The listing builds one solid part. Answer for the finished solid, in the listing's coordinates (mm). Round coordinates to 2 decimals unless told otherwise and drop trailing zeros. Write each loop counter-clockwise with the first axis right and the second up, starting at its lowest first coordinate (ties: lowest second). Pieces come first, ordered by that corner, then holes.
(1) Find the intervals of material crossed by probe 1 along X at (y, z) = (-106.5, 0.3); probe 2 along Y at (x, z) = (120, 1.25); probe 3 along X at (y, z) = (3.5, 0.4), in increasing order.
(2) A cutting plane is placed at A-A, the plane x = -2. Give the vertices of the cut face in (y, z).
(3) A cutting plane is placed at B-B, the plane z = 0.6. Give the number of separate pieces and of enclosed holes in the cut face, and give its area (3 significant figures).
Autodesk Inventor part; units mm, degrees
ref_plane "YZ Plane" through (0, 0, 0) normal (1, 0, 0) x (0, 1, 0)
ref_plane "XZ Plane" through (0, 0, 0) normal (0, 1, 0) x (-1, 0, 0)
ref_plane "XY Plane" through (0, 0, 0) normal (0, 0, 1) x (1, 0, 0)
sketch "Эскиз1" plane through (0, 0, 0) normal (0, 0, 1) x (1, 0, 0)
  line L0 (-145, 120) -> (145, 120)
  line L1 (145, 120) -> (145, -120)
  line L2 (145, -120) -> (-145, -120)
  line L3 (-145, -120) -> (-145, 120)
  line L4 (-145, 120) -> (145, -120) construction
  line L5 (145, 120) -> (-145, -120) construction
  point P0 (0, 0)
  dimension "d0" = 290
  dimension "d1" = 240
extrude "Выдавливание1" add sketch "Эскиз1" along normal blind 3
sketch "Эскиз2" plane through (0, 0, 3) normal (0, 0, 1) x (1, 0, 0)
  line L0 (-5, 95) -> (5, 95)
  line L1 (145, 120) -> (-145, 120)
  line L2 (0, 168) -> (0, -168)
  line L3 (-101.423, -89.3301) -> (-106.423, -80.6699)
  line L4 (106.423, -80.6699) -> (101.423, -89.3301)
  point P0 (0, 0)
  point P1 (0, 95)
  point P2 (0, -25)
  point P3 (-103.923, -85)
  point P4 (103.923, -85)
  dimension "d4" = 25
  dimension "d5" = 10
  dimension "d8" = 360
  dimension "d10" = 120
sketch "Эскиз4" plane through (0, 0, 0) normal (0, 0, -1) x (-1, 0, 0)
  line L0 (130, -15.5) -> (130, 9.5)
  line L1 (130, 9.5) -> (140, 9.5)
  line L2 (140, 9.5) -> (140, -15.5)
  line L3 (140, -15.5) -> (130, -15.5)
  line L4 (-15, -100) -> (15, -100)
  line L5 (15, -100) -> (15, -110)
  line L6 (15, -110) -> (-15, -110)
  line L7 (-15, -110) -> (-15, -100)
  line L8 (115, -100) -> (115, -110)
  line L9 (115, -110) -> (85, -110)
  line L10 (85, -110) -> (85, -100)
  line L11 (85, -100) -> (115, -100)
  line L12 (-130, -15.5) -> (-140, -15.5)
  line L13 (-140, -15.5) -> (-140, 9.5)
  line L14 (-140, 9.5) -> (-130, 9.5)
  line L15 (-130, 9.5) -> (-130, -15.5)
  circle A0 centre (120, 79) radius 1.5
  circle A1 centre (-120, -85) radius 1.5
  circle A2 centre (120, -85) radius 1.5
  line L16 (-85, -100) -> (-85, -110)
  line L17 (-85, -110) -> (-115, -110)
  line L18 (-115, -110) -> (-115, -100)
  line L19 (-115, -100) -> (-85, -100)
  circle A3 centre (-120, 79) radius 1.5
  line L20 (150, 119) -> (-150, 119)
  line L21 (-150, 119) -> (-150, -125)
  line L22 (-150, -125) -> (150, -125)
  line L23 (150, -125) -> (150, 119)
  point P0 (0, 0)
extrude "Выдавливание3" cut sketch "Эскиз4" against normal blind 10 contours L0 L1 L2 L3 | L4 L5 L6 L7 | L8 L9 L10 L11 | L12 L13 L14 L15 | A0 | A1 | A2 | L16 L17 L18 L19 | A3
sketch "Эскиз6" plane through (0, 0, 0) normal (0, 0, -1) x (-1, 0, 0)
  circle A0 centre (-115.363, -29) radius 2.5
  circle A1 centre (-115.363, 29) radius 2.5
  circle A2 centre (-74.363, 29) radius 2.5
  circle A3 centre (-74.363, -29) radius 2.5
  circle A4 centre (-25.5005, 12.1735) radius 1.0922
  circle A5 centre (-33.1205, 7.0935) radius 1.0922
  circle A6 centre (-25.5005, 12.1735) radius 1.0922
  circle A7 centre (16.1281, -25.2259) radius 1.5
  circle A8 centre (16.1281, -52.2259) radius 1.5
  circle A9 centre (-13.4032, -52.2259) radius 1.5
  circle A10 centre (-13.4032, -25.2259) radius 1.5
  circle A11 centre (66.1296, 35.3961) radius 1.5875
  circle A12 centre (66.1296, -47.1539) radius 1.5875
  circle A13 centre (114.3896, -40.8039) radius 1.5875
  circle A14 centre (99.1496, -16.6739) radius 1.5875
  circle A15 centre (71.2096, -16.6739) radius 1.5875
  circle A16 centre (114.3896, 34.1261) radius 1.5875
  line L0 (30, 37.5) -> (33, 37.5)
  line L1 (30, 34.5) -> (33, 34.5)
  line L2 (-33, 37.5) -> (-30, 37.5)
  line L3 (-33, 34.5) -> (-30, 34.5)
  line L4 (-33, 78.5) -> (-30, 78.5)
  line L5 (-33, 81.5) -> (-30, 81.5)
  line L6 (30, 78.5) -> (33, 78.5)
  line L7 (30, 81.5) -> (33, 81.5)
  circle A17 centre (31.5, 36) radius 1.5
  line L8 (33, 34.5) -> (33, 37.5) construction
  line L9 (-30, 34.5) -> (-30, 37.5) construction
  circle A18 centre (-31.5, 36) radius 1.5
  line L10 (33, 78.5) -> (33, 81.5) construction
  circle A19 centre (31.5, 80) radius 1.5
  circle A20 centre (-31.5, 80) radius 1.5
  line L11 (-33, 78.5) -> (-33, 81.5) construction
  point P0 (0, 0)
  dimension "d18" = 3
extrude "Выдавливание4" cut sketch "Эскиз6" against normal blind 10
sketch "Эскиз7" plane through (0, 0, 0) normal (0, 0, -1) x (-1, 0, 0)
  circle A0 centre (-95, 80) radius 1.5
  circle A1 centre (95, 80) radius 1.5
  circle A2 centre (95, -80) radius 1.5
  circle A3 centre (-95, -80) radius 1.5
  line L0 (-95, 80) -> (95, 80) construction
  line L1 (95, -80) -> (95, 80) construction
  circle A4 centre (-120, -85) radius 1.5 construction
  line L2 (-95, -80) -> (95, -80) construction
  line L3 (145, -120) -> (-145, -120) construction
  line L4 (-145, 120) -> (145, 120) construction
  line L5 (145, 120) -> (145, -120) construction
  line L6 (-95, 80) -> (-95, -80) construction
  line L7 (-145, -120) -> (-145, 120) construction
  point P0 (0, 0)
  dimension "d19" = 40
  dimension "d20" = 40
  dimension "d21" = 50
  dimension "d22" = 50
  dimension "d23" = 3
extrude "Выдавливание5" cut sketch "Эскиз7" against normal blind 10
properties part number "electronic_plate_long_side"
Solutions:
1. probe 1: x = -145 to -115, -85 to -15, 15 to 85, 115 to 145
1. probe 2: y = -120 to -86.5, -83.5 to 77.5, 80.5 to 120
1. probe 3: x = -145 to -140, -130 to 130, 140 to 145
2. outline: (-120, 0) - (-110, 0) - (-110, 3) - (-120, 3) - close; (-100, 0) - (120, 0) - (120, 3) - (-100, 3) - close
3. separate pieces: 1
3. enclosed holes: 33
3. area: 68,000 mm2
